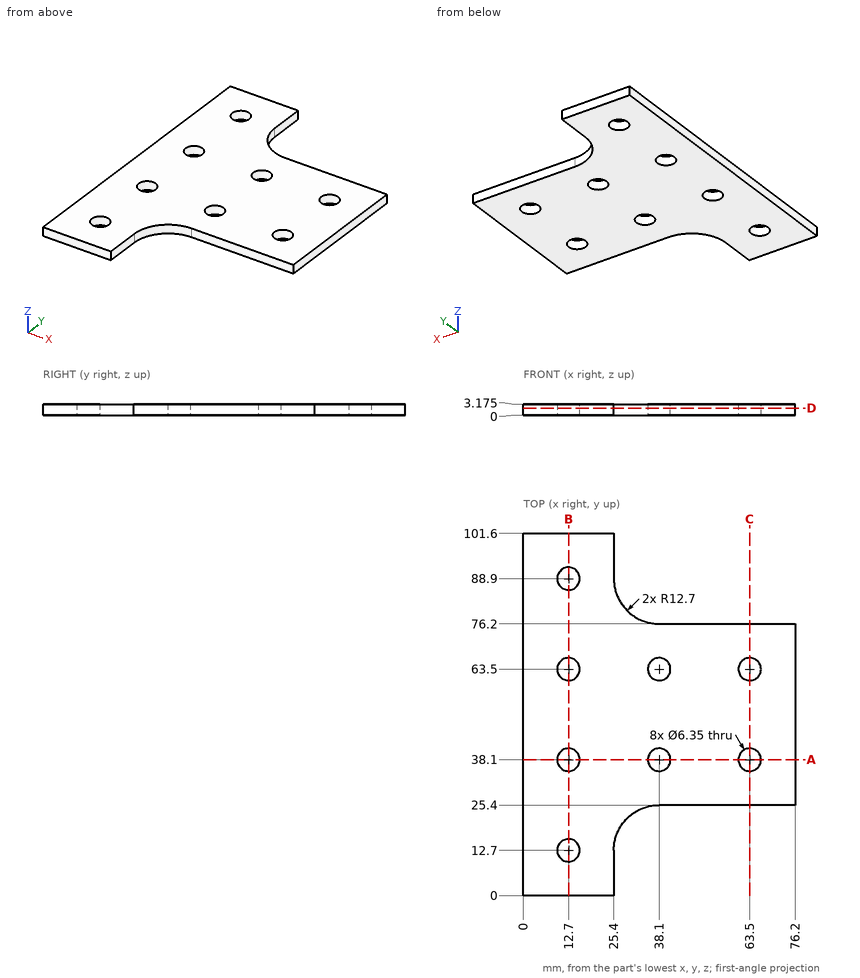
Part print with two shaded views. Sizes in mm from the minimum x, y, z corner. Coordinates: 2 decimals unless noted, no trailing zeros. Write each loop counter-clockwise with the first axis right and the second up, starting at its lowest first coordinate (ties: lowest second). Pieces come first, ordered by that corner, then holes.
(1) Cut at A-A on y = 38.1. List the corners of the cut face in (x, z) (3 decimals), and give its area (3 significant figures).
(2) Cut at B-B on x = 12.7. List the corners of the cut face in (y, z) (3 decimals), and give its area (3 significant figures).
(3) Drill centre lines: line 1 (Y direction, x = 12.7, z = 1.25) (3 decimals); line 2 (Y direction, x = 63.5, z = 1.85) (3 decimals); line 3 (Y direction, x = 37, z = 1.7). Where is each one in solid material? Low to high.
(4) Cut at D-D on z = 2. State how many separate pieces and enclosed holes the cut face has, and give its area (3 significant figures).
(5) Cut at C-C on x = 63.5. List the corners of the cut face in (y, z) (3 decimals).
(6) Pin check, flat tips, straight feed: pin 1 Ø4 at (x, y) = (63.5, 38.1) entering from -Z; pin 2 Ø1 at (x, z) = (54.5, 1) entering from +Y. Stop position of each tip, or through.
Working result:
1. outline: (0, 0) - (9.525, 0) - (9.525, 3.175) - (0, 3.175) - close; (15.875, 0) - (34.925, 0) - (34.925, 3.175) - (15.875, 3.175) - close; (41.275, 0) - (60.325, 0) - (60.325, 3.175) - (41.275, 3.175) - close; (66.675, 0) - (76.2, 0) - (76.2, 3.175) - (66.675, 3.175) - close
1. area: 181 mm2
2. outline: (0, 0) - (9.525, 0) - (9.525, 3.175) - (0, 3.175) - close; (15.875, 0) - (34.925, 0) - (34.925, 3.175) - (15.875, 3.175) - close; (41.275, 0) - (60.325, 0) - (60.325, 3.175) - (41.275, 3.175) - close; (66.675, 0) - (85.725, 0) - (85.725, 3.175) - (66.675, 3.175) - close; (92.075, 0) - (101.6, 0) - (101.6, 3.175) - (92.075, 3.175) - close
2. area: 242 mm2
3. line 1: y = 0 to 9.525, 15.875 to 34.925, 41.275 to 60.325, 66.675 to 85.725, 92.075 to 101.6
3. line 2: y = 25.4 to 34.925, 41.275 to 60.325, 66.675 to 76.2
3. line 3: y = 25.35 to 35.12, 41.08 to 60.52, 66.48 to 76.25
4. separate pieces: 1
4. enclosed holes: 8
4. area: 4,980 mm2
5. outline: (25.4, 0) - (34.925, 0) - (34.925, 3.175) - (25.4, 3.175) - close; (41.275, 0) - (60.325, 0) - (60.325, 3.175) - (41.275, 3.175) - close; (66.675, 0) - (76.2, 0) - (76.2, 3.175) - (66.675, 3.175) - close
6. pin 1: passes through
6. pin 2: stops at y = 76.2
